```python
from build123d import *

# Parameters (mm, degrees)
F1_DEPTH    = 25.4
F2_R        = 5.08
F3_R        = 5.08
F4_T1_DEPTH = 33.02
F4_S5_W     = 5.08
F4_S5_H     = 5.08
F4_T6_DEPTH = 5.08


# Not quite as in the source:
# - a fillet or chamfer that OpenCascade refuses, or shapes differently, is made with other operations: its cross-section is extruded or revolved along the edge and cut away or added


with BuildPart() as f1:
    # F0 (on Front) → F1 (new body)
    with BuildSketch(Plane.XZ):
        Polygon((0, -50.5684018135), (0, 52.7750141919), (-25.3761447966, 52.7750141919), (-25.3761447966, 23.721171543), (-11.0331093892, 23.721171543), (-11.0331093892, -10.1136825979), (-54.4299855828, -10.1136825979), (-54.4299855828, -50.5684018135), align=None)
    extrude(amount=F1_DEPTH)

    # F2
    f2_edges = [f1.edges().sort_by_distance(p)[0] for p in [
        (-12.688072, -25.4, 52.775014),
    ]]
    fillet(f2_edges, radius=F2_R)

    # F3
    f3_edges = [f1.edges().sort_by_distance(p)[0] for p in [
        (-27.214993, -25.4, -50.568402),
        (-54.429986, -25.4, -30.341042),
        (-32.731547, -25.4, -10.113683),
        (-11.033109, -25.4, 6.803744),
        (-25.376145, -25.4, 35.708093),
        (-18.204627, -25.4, 23.721172),
    ]]
    fillet(f3_edges, radius=F3_R)

    # F4: fillet of radius 5.08 on 1 edges, made by hand

    # F4_s2 → F4_t1 (cut)
    with BuildSketch(Plane.XZ.offset(-12.7)):
        with BuildLine():
            ThreePointArc((-54.4299855828, -15.1936825979), (-52.9420880313, -11.6015801494), (-49.3499855828, -10.1136825979))
            Line((-49.3499855828, -10.1136825979), (-54.4299855828, -10.1136825979))
            Line((-54.4299855828, -10.1136825979), (-54.4299855828, -15.1936825979))
        make_face()
    extrude(amount=F4_T1_DEPTH, mode=Mode.SUBTRACT)


with BuildPart() as f4_tool4:
    # F4_s5 → F4_t6 (new body)
    with BuildSketch(Plane.YZ.offset(-49.3499855828)):
        with Locations((-22.86, -12.6536825979)):
            Rectangle(F4_S5_W, F4_S5_H)
    extrude(amount=-F4_T6_DEPTH)

    # F4_s7 → F4_t8 (revolve, cut)
    with BuildSketch(Plane(origin=(-49.3499855828, -20.32, -15.1936825979), x_dir=(0, 0.7071067812, -0.7071067812), z_dir=(0, 0.7071067812, 0.7071067812))):
        with BuildLine():
            ThreePointArc((0, -5.08), (5.08, 0), (0, 5.08))
            Line((0, 5.08), (0, -5.08))
        make_face()
    revolve(axis=Axis((-49.3499855828, -20.32, -15.1936825979), (-1, 0, 0)), mode=Mode.SUBTRACT)


with BuildPart() as f1_1:
    add(f1.part)

    # F4_t3: cut F4_tool4
    add(f4_tool4.part, mode=Mode.SUBTRACT)


solid = f1_1.part
```
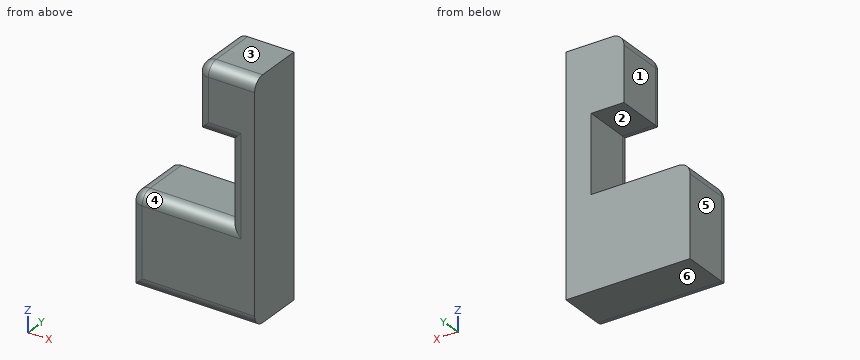
CAD build for the part. Positions are in the model's coordinates, mm. Face numbers are marked on the shaded views. A direction names the side the tool comes from. Round coordinates to 2 decimals unless told otherwise and drop trailing zeros. Order: outer loops, then holes, each group sorted by start corner. A loop starts at its lowest first (then second) coordinate and runs counter-clockwise, first axis right, second up.
Item 1: Saw through at A-A on x = -12. Write the cut outline in (y, z).
Item 2: Saw through at C-C on x = -30. Write the cut outline in (y, z).
Item 3: Pin check, flat tips, straight feed: pin 1 (2 mm diameter, centred on x = -24.5, y = -7.5, fed in from +Z); pin 2 (10 mm diameter, centred on y = -3.5, z = 29, fed in from -X); pin 3 (10 mm diameter, centred on x = -31, y = -12.5, fed in from +Z). Stop position of each tip, or through.
Item 4: Saw through at B-B on y = -18.5. Write the cut outline in (x, z).
Item 5: Probe line 1 along Z through (x, y) = (-37.5, -7); line 2 along X through (y, z) = (-20, 10); line 3 along Y through (x, z) = (-50, -42.5). List the from-to ranges inside material, lowest first.
Item 6: Tool access for the marked faces 1, 2 and 3: list every direction of +Z, -Z, +X, -X, +Y, -Y with a clear straight run to the whole face (end or side of a thin tool).
Item 7: Mould opens along Z. For the marked faces 4, 5 and 6 say: pulls with the +Z half, pulls with the -Z half, needs draft (parallel to the pull), parting line crosses it, or undercut.
Item 8: Saw through at D-D on z = 25. Write the cut outline in (x, y), then the cut area to 3 significant figures.
Reported:
1. outline: (-25.4, -45.49) arc R5.08 ccw to (-20.32, -50.57) - (0, -50.57) - (0, -10.11) - (-20.32, -10.11) arc R5.08 ccw to (-25.4, -15.19) - close; (-25.4, 28.8) arc R5.08 ccw to (-20.32, 23.72) - (0, 23.72) - (0, 52.78) - (-20.32, 52.78) arc R5.08 ccw to (-25.4, 47.7) - close
2. outline: (-25.4, -45.49) arc R5.08 ccw to (-20.32, -50.57) - (0, -50.57) - (0, -10.11) - (-20.32, -10.11) arc R5.08 ccw to (-25.4, -15.19) - close
3. pin 1: stops at z = 51.64
3. pin 2: stops at x = -25.38
3. pin 3: stops at z = -10.11
4. outline: (-54.43, -50.57) - (0, -50.57) - (0, 52.78) - (-20.3, 52.78) arc R5.08 ccw to (-25.38, 47.7) - (-25.38, 23.72) - (-11.03, 23.72) - (-11.03, -10.11) - (-49.35, -10.11) arc R5.08 ccw to (-54.43, -15.19) - close
5. line 1: z = -50.57 to -10.11
5. line 2: x = -11.03 to 0
5. line 3: y = -25.36 to 0
6. face 1: +Z, -X, +Y, -Y
6. face 2: -X, +Y, -Y
6. face 3: +Z, +X, -X, +Y, -Y
7. face 4: undercut
7. face 5: needs draft
7. face 6: pulls with the -Z half
8. outline: (-25.38, -20.32) arc R5.08 ccw to (-24.1, -23.69) - (-9.75, -23.69) arc R5.08 ccw to (-5.95, -25.4) - (0, -25.4) - (0, 0) - (-25.38, 0) - close
8. area: 614 mm2
